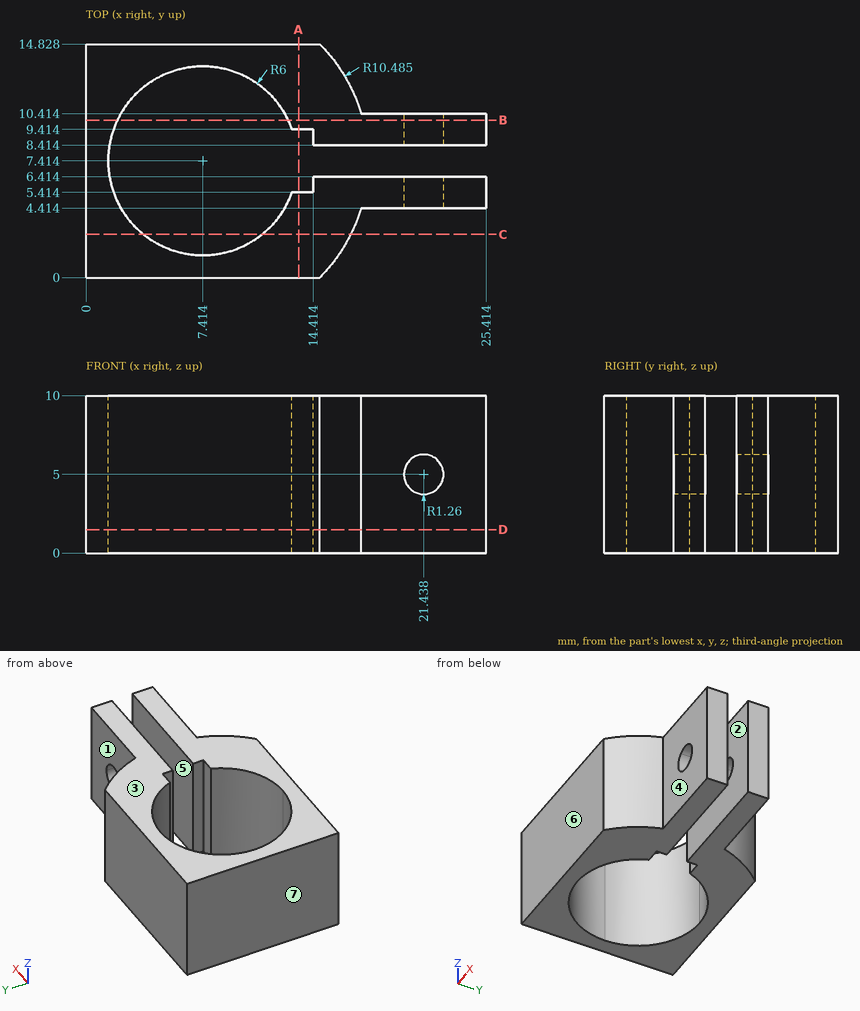
Geometry check sheet. Reference: drawing and pictorial views, mm from the part's lowest x, y, z. A direction names the side the tool comes from. Give positions to 0.01 mm unless a question says otherwise; leave off trailing zeros. Loops run counter-clockwise (first coordinate to the right, second up) from the corner with the lowest first, then second, coordinate; pieces in that order, holes last. Notation, with made-up numbers: M 5.5,83 L 23.5,83 A19 cw 23.5,99 Z; hole C -14,64 d7. An arc over 180 degrees is marked long. One line per question, with ' | ' between items.
Item 1: Section check A-A, the plane x = 13.5. Record the cut outline in (y, z) (1 decimal).
Completed:
outline: M 0,0 L 5.4,0 L 5.4,10 L 0,10 Z; M 9.4,0 L 14.8,0 L 14.8,10 L 9.4,10 Z
Item 2: Section check B-B, the plane y = 10. Record the cut outline in (x, z) (1 decimal), plus the area to 3 significant figures.
Completed:
outline: M 0,0 L 2,0 L 2,10 L 0,10 Z; M 12.8,0 L 25.4,0 L 25.4,10 L 12.8,10 Z; hole C 21.4,5 d2.5 | area: 141 mm^2
Item 3: Section check C-C, the plane y = 2.75. Record the cut outline in (x, z) (1 decimal).
Completed:
outline: M 0,0 L 3.6,0 L 3.6,10 L 0,10 Z; M 11.2,0 L 16.8,0 L 16.8,10 L 11.2,10 Z
Item 4: Draft check along Y on the marked faces 5, 6 and 7. Enter one of: +Y half, -Y half, draft (parallel to the pull), parting line (faces both ways), or undercut.
Completed:
face 5: undercut | face 6: -Y half | face 7: draft
Item 5: Thickness scan on line 1 (Y direction, x = 17.5, z = 1) (1 decimal); line 2 (Y direction, x = 7.25, z = 5); line 3 (X direction, y = 10.5, z = 8.5) (1 decimal). Record the ranges inside material, lowest first. Write a range as [from, to].
Completed:
line 1: y = [4.4, 6.4], [8.4, 10.4] | line 2: y = [0, 1.42], [13.41, 14.83] | line 3: x = [0, 2.3], [12.6, 17.4]
Item 6: Section check D-D, the plane z = 1.5. Record the cut outline in (x, y) (1 decimal), plus the area to 3 significant figures.
Completed:
outline: M 0,0 L 14.8,0 A10.5 ccw 17.5,4.4 L 25.4,4.4 L 25.4,6.4 L 14.4,6.4 L 14.4,5.4 L 13.1,5.4 A6 cw long 13.1,9.4 L 14.4,9.4 L 14.4,8.4 L 25.4,8.4 L 25.4,10.4 L 17.5,10.4 A10.5 ccw 14.8,14.8 L 0,14.8 Z | area: 158 mm^2
Item 7: Depth check by flat-ended pin: P1, Ø2, axis at y = 8.5, z = 3, coming from the -X side; P2, Ø5, axis at x = 21.5, z = 3.5, coming from the -Y side; P3, Ø3, axis at x = 6.5, y = 11, coming from the -Z side; P4, Ø3, axis at x = 19, z = 5.5, coming from the +Y side. Enter the tip coordinate at first touch or a pass-through.
Completed:
P1: stops at x = 0 | P2: stops at y = 4.41 | P3: passes through | P4: stops at y = 10.41
Item 8: Tool access check on the marked faces 1, 2, 3 and 4. Record the directions out of +Z, -Z, +X, -X, +Y, -Y that give a thin tool (end or side, any length) a straight path to the whole face; none if there is none.
Completed:
face 1: +Z, -Z, +X, +Y | face 2: +Z, -Z, +X | face 3: +Z, +X, -X, +Y, -Y | face 4: +Z, -Z, +X, -Y
